```python
from build123d import *

# Parameters (mm, degrees)
BASPROSKE_W        = 12
BASPROSKE_H        = 24
TOOTHCUT_DEPTH     = 37
TEETHCUTS_COUNT    = 22
TEETHCUTS_ANGLE    = 343.636363636
BORSKE_R           = 3
BORE_DEPTH         = 50.0000508
SKETCH1_R          = 10
CUT_EXTRUDE1_DEPTH = 4.5
CUT_EXTRUDE2_REACH = 36.656
SKETCH2_R          = 3.5
CUT_EXTRUDE3_REACH = 36.656
SKETCH3_R          = 1.325


with BuildPart() as part:
    # BasProSke → Base-Revolve (revolve)
    with BuildSketch(Plane(origin=(0, 0, 0), x_dir=(1, 0, 0), z_dir=(0, 1, 0)), mode=Mode.PRIVATE) as base_revolve_sk:
        with Locations((6, 12)):
            Rectangle(BASPROSKE_W, BASPROSKE_H)
    revolve(base_revolve_sk.sketch.rotate(Axis((-10, 0, 0), (1, 0, 0)), 180), axis=Axis((-10, 0, 0), (1, 0, 0)))

    # TooCutSke → ToothCut (cut, through all)
    with BuildSketch(Plane(origin=(0, 0, 0), x_dir=(0, 0, -1), z_dir=(1, 0, 0))):
        with BuildLine():
            ThreePointArc((1.148067356, 19.465172549), (0, 19.499), (-1.148067356, 19.465172549))
            ThreePointArc((-1.148067356, 19.465172549), (-1.628029232, 21.774154728), (-2.703966408, 23.872754571))
            ThreePointArc((-2.703966408, 23.872754571), (0, 24.0254), (2.703966408, 23.872754571))
            ThreePointArc((2.703966408, 23.872754571), (1.628029232, 21.774154728), (1.148067356, 19.465172549))
        make_face()
    toothcut = extrude(amount=TOOTHCUT_DEPTH, mode=Mode.SUBTRACT)

    # TeethCuts: ToothCut ×22 about axis
    teethcuts_axis = Axis((-10, 0, 0), (1, 0, 0))
    for i in range(1, TEETHCUTS_COUNT):
        add(toothcut.rotate(teethcuts_axis, i * TEETHCUTS_ANGLE / (TEETHCUTS_COUNT - 1)), mode=Mode.SUBTRACT)

    # BorSke → Bore (cut, symmetric)
    with BuildSketch(Plane(origin=(0, 0, 0), x_dir=(0, 0, -1), z_dir=(1, 0, 0))):
        with Locations(Location((0, 0, 0), (0, 0, 180))):
            Circle(BORSKE_R)
    extrude(amount=BORE_DEPTH, both=True, mode=Mode.SUBTRACT)

    # Sketch1 → Cut-Extrude1 (cut)
    with BuildSketch(Plane(origin=(12, 0, 0), x_dir=(0, 0, -1), z_dir=(1, 0, 0))):
        Circle(SKETCH1_R)
    extrude(amount=-CUT_EXTRUDE1_DEPTH, mode=Mode.SUBTRACT)

    # Sketch2 → Cut-Extrude2 (cut, up to next)
    with BuildSketch(Plane(origin=(7.5, 0, 0), x_dir=(0, 0, -1), z_dir=(1, 0, 0)), mode=Mode.PRIVATE) as cut_extrude2_sk1:
        Circle(SKETCH2_R)
    cut_extrude2_tool1 = extrude(cut_extrude2_sk1.sketch, amount=-CUT_EXTRUDE2_REACH, mode=Mode.PRIVATE) & part.part
    add(cut_extrude2_tool1.solids().sort_by_distance((7.5, 0, 0))[0], mode=Mode.SUBTRACT)

    # Sketch3 → Cut-Extrude3 (cut, up to next)
    with BuildSketch(Plane(origin=(7.5, 0, 0), x_dir=(0, 0, -1), z_dir=(1, 0, 0)), mode=Mode.PRIVATE) as cut_extrude3_sk1:
        with Locations((0, 7)):
            Circle(SKETCH3_R)
    cut_extrude3_tool1 = extrude(cut_extrude3_sk1.sketch, amount=-CUT_EXTRUDE3_REACH, mode=Mode.PRIVATE) & part.part
    # Sketch3 → Cut-Extrude3 (cut, up to next)
    with BuildSketch(Plane(origin=(7.5, 0, 0), x_dir=(0, 0, -1), z_dir=(1, 0, 0)), mode=Mode.PRIVATE) as cut_extrude3_sk2:
        with Locations((7, 0)):
            Circle(SKETCH3_R)
    cut_extrude3_tool2 = extrude(cut_extrude3_sk2.sketch, amount=-CUT_EXTRUDE3_REACH, mode=Mode.PRIVATE) & part.part
    # Sketch3 → Cut-Extrude3 (cut, up to next)
    with BuildSketch(Plane(origin=(7.5, 0, 0), x_dir=(0, 0, -1), z_dir=(1, 0, 0)), mode=Mode.PRIVATE) as cut_extrude3_sk3:
        with Locations((0, -7)):
            Circle(SKETCH3_R)
    cut_extrude3_tool3 = extrude(cut_extrude3_sk3.sketch, amount=-CUT_EXTRUDE3_REACH, mode=Mode.PRIVATE) & part.part
    # Sketch3 → Cut-Extrude3 (cut, up to next)
    with BuildSketch(Plane(origin=(7.5, 0, 0), x_dir=(0, 0, -1), z_dir=(1, 0, 0)), mode=Mode.PRIVATE) as cut_extrude3_sk4:
        with Locations((-7, 0)):
            Circle(SKETCH3_R)
    cut_extrude3_tool4 = extrude(cut_extrude3_sk4.sketch, amount=-CUT_EXTRUDE3_REACH, mode=Mode.PRIVATE) & part.part
    add(cut_extrude3_tool1.solids().sort_by_distance((7.5, 7, 0))[0], mode=Mode.SUBTRACT)
    add(cut_extrude3_tool2.solids().sort_by_distance((7.5, 0, -7))[0], mode=Mode.SUBTRACT)
    add(cut_extrude3_tool3.solids().sort_by_distance((7.5, -7, 0))[0], mode=Mode.SUBTRACT)
    add(cut_extrude3_tool4.solids().sort_by_distance((7.5, 0, 7))[0], mode=Mode.SUBTRACT)


solid = part.part
```
Input: part model. Units: mm. Frame: model coordinates. A direction names the side the tool comes from. Coordinates: 2 decimals unless noted, no trailing zeros. Loops run counter-clockwise (first coordinate to the right, second up) from the corner with the lowest first, then second, coordinate; pieces in that order, holes last. Notation, with made-up numbers: M 2.25,1.25 L 23.25,1.25 A28 ccw 23.25,33.25 Z; hole C 1.25,58.25 d8. An arc over 180 degrees is marked long. Use a Markdown table: item, result. Add a question column.
1) Section A-A, the plane z = 0. Return the cut outline in (x, y) (3 decimals), plus the area to 3 significant figures.
2) Pin query (flat end, axial travel): P1, Ø5, axis at x = 1, y = -4, coming from the +Z side; P2, Ø4, axis at x = 4, z = 9.5, coming from the -Y side; P3, Ø2, axis at x = 3, y = 19, coming from the -Z side. Return the tip coordinate at first contact, or that it passes through.
3) Line query: L1, parallel to Y at x = 11.25, z = 22; L2, parallel to Z at x = 11.75, y = 12; L3, parallel to Y at x = 10, z = -4. Output: solid intervals per line, ascending. Write a range as from..to.
4) Section C-C, the plane x = 2.5. Give the number of separate pieces and of enclosed holes in the cut face, plus the area to 3 significant figures.
5) Draft query along Z for faces 5 (the cylindrical face through (6.084, 23.757, 3.405)), 6 (the cylindrical face through (3.802, 0.398, -8.264)), 7 (the cylindrical face through (6.084, -12.984, -20.185)). Return one class per face: +Z half, -Z half, draft (parallel to the pull), parting line (faces both ways), or undercut.
6) Section B-B, the plane y = 4.5. Return the cut outline in (x, z).
7) Set-up query: faces 1 (the cylindrical face through (5.92, -17.45, 13.16)), 2 (the cylindrical face through (5.916, -12.781, -14.726)), 3 (the cylindrical face through (5.92, 15.51, 15.4)), 4 (the cylindrical face through (5.9, -10.5, -19.1)). Return all of +Z, -Z, +X, -X, +Y, -Y with unobstructed straight access to the full face (end or side cutting, diameter ignored); none if empty.
Answer below:
| question | item | result |
|---|---|---|
| 1 | outline | M 0,-19.499 L 12,-19.499 L 12,-10 L 7.5,-10 L 7.5,-8.325 L 0,-8.325 Z; M 0,-5.675 L 7.5,-5.675 L 7.5,-3.5 L 0,-3.5 Z; M 0,3.5 L 7.5,3.5 L 7.5,5.675 L 0,5.675 Z; M 0,8.325 L 7.5,8.325 L 7.5,10 L 12,10 L 12,19.499 L 0,19.499 Z |
| 1 | area | 286 mm2 |
| 2 | P1 | z = 23.22 |
| 2 | P2 | y = -22.13 |
| 2 | P3 | z = -15.87 |
| 3 | L1 | -7.57..-5.11, -1.44..1.44, 5.11..7.57 |
| 3 | L2 | -20.36..-15.63, -15.37..15.37, 15.63..20.36 |
| 3 | L3 | -23.66..-9.17, 9.17..23.66 |
| 4 | separate pieces | 1 |
| 4 | enclosed holes | 5 |
| 4 | area | 1,410 mm2 |
| 5 | face 5 | +Z half |
| 5 | face 6 | undercut |
| 5 | face 7 | -Z half |
| 6 | outline | M 0,-20.89 L 12,-20.89 L 12,-8.93 L 7.5,-8.93 L 7.5,8.93 L 12,8.93 L 12,20.89 L 0,20.89 Z |
| 7 | face 1 | +X, -X, -Y |
| 7 | face 2 | +X, -X |
| 7 | face 3 | +Z, +X, -X |
| 7 | face 4 | -Z, +X, -X |
